For this review, take the finished solid that the model builds, in its own axes (mm). Give positions to 0.01 mm unless a question says otherwise; leave off trailing zeros. Loops run counter-clockwise (first coordinate to the right, second up) from the corner with the lowest first, then second, coordinate; pieces in that order, holes last.
```python
from build123d import *

# Parameters (mm, degrees)
SKETCH1_W           = 29.6
SKETCH1_H           = 10
BOSS_EXTRUDE1_DEPTH = 8
SKETCH2_R           = 4.8
CUT_EXTRUDE1_DEPTH  = 10
SKETCH4_R           = 1.6
CUT_EXTRUDE2_DEPTH  = 8
SKETCH7_R           = 1.6
CUT_EXTRUDE3_DEPTH  = 8


with BuildPart() as part:
    # Sketch1 → Boss-Extrude1 (new body)
    with BuildSketch(Plane(origin=(0, 0, 0), x_dir=(1, 0, 0), z_dir=(0, 1, 0))):
        with Locations((-14.8, 5)):
            Rectangle(SKETCH1_W, SKETCH1_H)
    extrude(amount=BOSS_EXTRUDE1_DEPTH)

    # Sketch2 → Cut-Extrude1 (cut)
    with BuildSketch(Plane.XY):
        with Locations((-14.8, 0)):
            Circle(SKETCH2_R)
    extrude(amount=-CUT_EXTRUDE1_DEPTH, mode=Mode.SUBTRACT)

    # Sketch4 → Cut-Extrude2 (cut)
    with BuildSketch(Plane.XZ):
        with Locations((-24.6, -5)):
            Circle(SKETCH4_R)
    extrude(amount=-CUT_EXTRUDE2_DEPTH, mode=Mode.SUBTRACT)

    # Sketch7 → Cut-Extrude3 (cut)
    with BuildSketch(Plane.XZ):
        with Locations((-5, -5)):
            Circle(SKETCH7_R)
    extrude(amount=-CUT_EXTRUDE3_DEPTH, mode=Mode.SUBTRACT)


solid = part.part
```
Q1. Mouldability with a two-part tool opening along X and no side actions: class faces 1 (the cylindrical face through (-6.6, 3.94, -4.93)), 2 (the flat face through (0, 4, -5)), 3 (the flat face through (-15, 5, 0)) as +X half, -X half, draft (parallel to the pull), parting line (faces both ways), or undercut.
Answers:
face 1: undercut
face 2: +X half
face 3: draft
Q2. For pin 1 Ø2 at (x, z) = (-18, -6.5) entering from -Y, flat-tipped, find the tip position at first contact; note if it passes through.
Answers:
pin 1: stops at y = 2.32
Q3. For probe 1 along Z at (x, y) = (-24.6, 5.75); probe 2 along X at (y, z) = (5.75, -5.75); probe 3 along X at (y, z) = (4, -5.5), list the stretches that pass through material, from the lowest coordinate up.
Answers:
probe 1: z = -10 to -6.6, -3.4 to 0
probe 2: x = -29.6 to -26.01, -23.19 to -6.41, -3.59 to 0
probe 3: x = -29.6 to -26.12, -23.08 to -17.45, -12.15 to -6.52, -3.48 to 0
Q4. Consider section A-A on z = -5. Give the boundary of the cut face in (x, y).
Answers:
outline: (-29.6, 0) - (-26.2, 0) - (-26.2, 8) - (-29.6, 8) - close; (-23, 0) - (-19.6, 0) arc R4.8 cw to (-10, 0) - (-6.6, 0) - (-6.6, 8) - (-23, 8) - close; (-3.4, 0) - (0, 0) - (0, 8) - (-3.4, 8) - close
Q5. Consider section D-D on y = 5.5. Give the boundary of the cut face in (x, z), plus the area to 3 significant figures.
Answers:
outline: (-29.6, -10) - (0, -10) - (0, 0) - (-29.6, 0) - close; hole circle Ø3.2 at (-24.6, -5); hole circle Ø3.2 at (-5, -5)
area: 280 mm2
Q6. Consider section B-B on y = 3. Give the boundary of the cut face in (x, z), plus the area to 3 significant figures.
Answers:
outline: (-29.6, -10) - (-18.55, -10) - (-18.55, 0) - (-29.6, 0) - close; (-11.05, -10) - (0, -10) - (0, 0) - (-11.05, 0) - close; hole circle Ø3.2 at (-24.6, -5); hole circle Ø3.2 at (-5, -5)
area: 205 mm2
Q7. Consider section C-C on x = -5. Give the boundary of the cut face in (y, z), plus the area to 3 significant figures.
Answers:
outline: (0, -10) - (8, -10) - (8, -6.6) - (0, -6.6) - close; (0, -3.4) - (8, -3.4) - (8, 0) - (0, 0) - close
area: 54.4 mm2
